Autodesk Inventor part; units mm, degrees
ref_plane "YZ Plane" through (0, 0, 0) normal (1, 0, 0) x (0, 1, 0)
ref_plane "XZ Plane" through (0, 0, 0) normal (0, 1, 0) x (-1, 0, 0)
ref_plane "XY Plane" through (0, 0, 0) normal (0, 0, 1) x (1, 0, 0)
sketch "Sketch1" plane through (0, 0, 0) normal (0, 0, 1) x (1, 0, 0)
  line L0 (9.7407, 1114.2593) -> (159.7407, 1114.2593)
  line L1 (9.7407, 1114.2593) -> (-140.2593, 1114.2593)
  line L2 (-290.2593, 814.2593) -> (-140.2593, 1114.2593)
  line L3 (159.7407, 1114.2593) -> (459.7407, 514.2593)
  line L4 (135.0194, 1074.2593) -> (9.7407, 1074.2593)
  line L5 (9.7407, 1074.2593) -> (-115.5379, 1074.2593)
  line L6 (-115.5379, 1074.2593) -> (-245.5379, 814.2593)
  line L7 (9.7407, 1114.2593) -> (159.7407, 1114.2593)
  line L8 (9.7407, 1114.2593) -> (-140.2593, 1114.2593)
  line L9 (-440.2593, 514.2593) -> (-140.2593, 1114.2593)
  line L10 (159.7407, 1114.2593) -> (309.9483, 813.8441)
  line L11 (135.0194, 1074.2593) -> (9.7407, 1074.2593)
  line L12 (9.7407, 1074.2593) -> (-115.5379, 1074.2593)
  line L13 (-115.5379, 1074.2593) -> (-245.5379, 814.2593)
  line L14 (-245.5379, 814.2593) -> (-290.2593, 814.2593)
  line L15 (265.227, 813.8441) -> (309.9483, 813.8441)
  line L16 (265.227, 813.8441) -> (135.0194, 1074.2593)
  line L17 (415.0194, 514.2593) -> (135.0194, 1074.2593)
  line L18 (-395.5379, 514.2593) -> (-440.2593, 514.2593)
  line L19 (-245.5379, 814.2593) -> (-395.5379, 514.2593)
  line L20 (-440.2593, 514.2593) -> (-395.5379, 514.2593)
  line L21 (415.0194, 514.2593) -> (459.7407, 514.2593)
  point P0 (0, 0)
  dimension "d13" = 300
extrude "Extrusion1" add sketch "Sketch1" along normal blind 40 contours L0 L3 L15 L16 L4 L5 L6 L14 L2 L1
fillet "Fillet2" radius 0.5 1 edges at (200.1232, 944.0517, 0)
fillet "Fillet3" radius 0.5 3 edges at (159.7407, 1114.2593, 20) (84.7407, 1114.2593, 0) (-215.2593, 964.2593, 0)
sketch "Sketch2" plane through (-140.2593, 1114.2593, 0.5) normal (0, 1, 0) x (1, 0, 0)
  line L0 (300.1382, -39.5) -> (300.1382, 0.4472)
  line L1 (300.1382, -19.5) -> (0, -19.5)
  line L2 (0, 0) -> (0, -39.5)
  circle A0 centre (150.0691, -19.5) radius 1.5
  point P0 (140.2593, 0.5)
  point P1 (300.1382, -39)
  point P2 (300.1382, 0)
  point P3 (0, -39)
  dimension "d14" = 3
extrude "Extrusion2" cut sketch "Sketch2" against normal blind 10
extrude "Extrusion3" add sketch "Sketch1" along normal blind 40 contours L3 L21 L17 L15 | L14 L19 L18 L9
sketch "Sketch3" plane through (-140.2593, 1114.2593, 0.5) normal (0, 1, 0) x (1, 0, 0)
  point P0 (140.2593, 0.5)
sketch "Sketch4" plane through (-140.2593, 1114.2593, 0.5) normal (0, 1, 0) x (1, 0, 0)
  circle A0 centre (150.0691, -19.5) radius 1.5
  line L0 (0, 0) -> (299.691, 0)
  line L1 (0, 0) -> (0, -39.5)
  line L2 (299.691, 0) -> (299.691, -39.5)
  line L3 (200.1691, -14.5) -> (225.9691, -14.5)
  line L4 (225.9691, -24.5) -> (200.1691, -24.5)
  arc A1 (225.9691, -24.5) -> (225.9691, -14.5) centre (225.9691, -19.5) ccw
  arc A2 (200.1691, -14.5) -> (200.1691, -24.5) centre (200.1691, -19.5) ccw
  arc A3 (74.1691, -14.5) -> (74.1691, -24.5) centre (74.1691, -19.5) ccw
  line L5 (74.1691, -14.5) -> (99.9691, -14.5)
  line L6 (74.1691, -24.5) -> (99.9691, -24.5)
  arc A4 (99.9691, -24.5) -> (99.9691, -14.5) centre (99.9691, -19.5) ccw
  line L7 (299.691, -39.5) -> (0, -39.5)
  point P0 (140.2593, 0.5)
extrude "Extrusion4" cut sketch "Sketch4" against normal blind 50 contours L3 A1 L4 A2 | L5 A4 L6 A3
sketch "Esboço5" plane through (0, 0, 0) normal (0, 0, 1) x (1, 0, 0)
  line L0 (159.4317, 1114.2593) -> (-140.2593, 1114.2593)
  line L1 (-94.9789, 1114.2593) -> (-94.9789, 897.5465)
  line L2 (-94.9789, 897.5465) -> (-260.935, 897.5465)
  line L3 (-290.2593, 814.2593) -> (-140.2593, 1114.2593)
  line L4 (-250.2227, 877.5465) -> (-250.2227, 857.5465)
  line L5 (265.227, 813.8441) -> (135.0194, 1074.2593)
  line L6 (223.3758, 897.5465) -> (233.3758, 897.5465)
  line L7 (233.3758, 897.5465) -> (233.3758, 882.5465)
  line L8 (-94.9789, 897.5465) -> (445.9224, 897.5465)
  line L9 (268.1798, 897.5465) -> (258.1798, 897.5465)
  line L10 (268.1798, 897.5465) -> (258.1798, 897.5465)
  line L11 (258.1798, 897.5465) -> (258.1798, 882.5465)
  line L12 (258.1798, 882.5465) -> (258.1798, 877.5465)
  line L13 (258.1798, 862.5465) -> (258.1798, 857.5465)
  line L14 (258.1798, 857.5465) -> (258.1798, 852.5465)
  arc A0 (253.1798, 857.5465) -> (263.1798, 857.5465) centre (258.1798, 857.5465) ccw
  arc A1 (263.1798, 877.5465) -> (253.1798, 877.5465) centre (258.1798, 877.5465) ccw
  line L15 (263.1798, 877.5465) -> (263.1798, 857.5465)
  line L16 (253.1798, 857.5465) -> (253.1798, 877.5465)
  line L17 (-248.6157, 897.5465) -> (-293.337, 808.1037)
  line L18 (268.1798, 897.5465) -> (312.835, 808.0707)
  line L19 (459.7407, 514.2593) -> (159.9907, 1113.7593)
  line L20 (-293.337, 808.1037) -> (-248.6157, 808.1037)
  line L21 (-395.5379, 514.2593) -> (-115.5379, 1074.2593)
  line L22 (-248.6157, 808.1037) -> (-258.6157, 808.1037)
  line L23 (-258.6157, 808.1037) -> (-258.6157, 823.1037)
  line L24 (-258.6157, 823.1037) -> (-258.6157, 828.1037)
  line L25 (-258.6157, 848.1037) -> (-258.6157, 853.1037)
  arc A2 (-253.6157, 848.1037) -> (-263.6157, 848.1037) centre (-258.6157, 848.1037) ccw
  arc A3 (-263.6157, 828.1037) -> (-253.6157, 828.1037) centre (-258.6157, 828.1037) ccw
  line L26 (-263.6157, 828.1037) -> (-263.6157, 848.1037)
  line L27 (-253.6157, 848.1037) -> (-253.6157, 828.1037)
  line L28 (-258.6157, 828.1037) -> (-258.6157, 833.1037)
  line L29 (-258.6157, 843.1037) -> (-258.6157, 848.1037)
  line L30 (312.835, 808.0707) -> (268.1137, 808.0707)
  line L31 (135.0194, 1074.2593) -> (415.0194, 514.2593)
  line L32 (268.1137, 808.0707) -> (278.1137, 808.0707)
  line L33 (278.1137, 808.0707) -> (278.1137, 823.0707)
  line L34 (278.1137, 823.0707) -> (278.1137, 828.0707)
  line L35 (278.1137, 848.0707) -> (278.1137, 853.0707)
  arc A4 (283.1137, 848.0707) -> (273.1137, 848.0707) centre (278.1137, 848.0707) ccw
  arc A5 (273.1137, 828.0707) -> (283.1137, 828.0707) centre (278.1137, 828.0707) ccw
  line L36 (273.1137, 848.0707) -> (273.1137, 828.0707)
  line L37 (283.1137, 848.0707) -> (283.1137, 828.0707)
  line L38 (278.1137, 828.0707) -> (278.1137, 833.0707)
  line L39 (278.1137, 843.0707) -> (278.1137, 848.0707)
  line L40 (-238.6157, 882.5465) -> (-238.6157, 862.5465)
  line L41 (-233.6157, 862.5465) -> (-233.6157, 882.5465)
  line L42 (-243.6157, 882.5465) -> (-243.6157, 862.5465)
  line L43 (-248.6157, 897.5465) -> (-238.6157, 897.5465)
  line L44 (-238.6157, 897.5465) -> (-238.6157, 882.5465)
  line L45 (-293.337, 808.1037) -> (-248.6157, 808.1037)
  line L46 (-248.6157, 897.5465) -> (-238.6157, 897.5465)
  line L47 (-238.6157, 897.5465) -> (-238.6157, 882.5465)
  line L48 (-238.6157, 882.5465) -> (-238.6157, 877.5465)
  line L49 (-238.6157, 857.5465) -> (-238.6157, 852.5465)
  arc A6 (-243.6157, 857.5465) -> (-233.6157, 857.5465) centre (-238.6157, 857.5465) ccw
  arc A7 (-233.6157, 877.5465) -> (-243.6157, 877.5465) centre (-238.6157, 877.5465) ccw
  line L50 (-243.6157, 877.5465) -> (-243.6157, 857.5465)
  line L51 (-233.6157, 857.5465) -> (-233.6157, 877.5465)
  line L52 (-238.6157, 877.5465) -> (-238.6157, 872.5465)
  line L53 (-238.6157, 862.5465) -> (-238.6157, 857.5465)
  point P0 (0, 0)
  dimension "d23" = 216.7128
  dimension "d33" = 10
  dimension "d34" = 15
  dimension "d35" = 5
  dimension "d37" = 20
  dimension "d38" = 5
  dimension "d39" = 10
  dimension "d40" = 100
  dimension "d41" = 100
  dimension "d42" = 10
  dimension "d43" = 15
  dimension "d44" = 5
  dimension "d45" = 20
  dimension "d46" = 5
  dimension "d47" = 10
  dimension "d48" = 10
  dimension "d49" = 10
  dimension "d50" = 15
  dimension "d51" = 5
  dimension "d52" = 20
  dimension "d53" = 5
  dimension "d54" = 10
  dimension "d55" = 10
  dimension "d69" = 10
  dimension "d70" = 15
  dimension "d71" = 5
  dimension "d72" = 20
  dimension "d73" = 5
  dimension "d74" = 10
  dimension "d75" = 10
extrude "Extrusão5" cut sketch "Esboço5" along normal mid plane 1000 contours A5 L36 A4 L37 | A1 L15 A0 L16 | A3 L26 A2 L27 | A7 L41 L51 A6 L49 L53 L40 | L40 L53 L49 A6 L50 L42 A7
sketch "Esboço8" plane through (0, 0, 40) normal (0, 0, 1) x (1, 0, 0)
  point P0 (0, 0)
properties part number "Cavalete_Inferior" material "SAE 1010/1020"
Build history of the part. All positions in model axes, mm. A direction names the side the tool comes from. Coordinates: 2 decimals unless noted, no trailing zeros. Order: outer loops, then holes, each group sorted by start corner. A loop starts at its lowest first (then second) coordinate and runs counter-clockwise, first axis right, second up. Notation, with made-up numbers: (54.5, 34) - (68.5, 34) arc R6 cw to (68.5, 42) - close; hole circle Ø1 at (75, 25). An arc over 180 degrees is marked (long way). Put each result on its own line as item: value.
1. Saw through at A-A (z = 31.5). Write the cut outline in (x, y), and give its area (3 significant figures).
Answer sheet:
outline: (-440.26, 514.26) - (-395.54, 514.26) - (-115.54, 1074.26) - (135.02, 1074.26) - (415.02, 514.26) - (459.74, 514.26) - (159.88, 1113.98) arc R0.5 ccw to (159.43, 1114.26) - (-140.26, 1114.26) - close; hole (-263.62, 828.1) arc R5 ccw to (-253.62, 828.1) - (-253.62, 848.1) arc R5 ccw to (-263.62, 848.1) - close; hole (-243.62, 857.55) arc R5 ccw to (-233.62, 857.55) - (-233.62, 877.55) arc R5 ccw to (-243.62, 877.55) - close; hole (253.18, 857.55) arc R5 ccw to (263.18, 857.55) - (263.18, 877.55) arc R5 ccw to (253.18, 877.55) - close; hole (273.11, 828.07) arc R5 ccw to (283.11, 828.07) - (283.11, 848.07) arc R5 ccw to (273.11, 848.07) - close
area: 61,800 mm^2
2. Drop flat-ended pins along their axis: P1, Ø22, axis at y = 836, z = 25, coming from the -X side; P2, Ø1, axis at y = 955, z = 15, coming from the -X side; P3, Ø0.6, axis at x = 265.5, z = 0, coming from the +Y side. Give the stop position or say it passes through.
Answer sheet:
P1: stops at x = -284.89
P2: stops at x = -220.14
P3: stops at y = 903.34
3. Probe line 1 along X through (y, z) = (1111.5, 20); line 2 along X through (y, z) = (869.5, 15.5); line 3 along X through (y, z) = (694, 23.5). List the from-to ranges inside material, lowest first. Write a range as [from, to].
Answer sheet:
line 1: x = [-141.64, -71.09], [-35.29, 8.31], [11.31, 54.91], [90.71, 161.12]
line 2: x = [-262.64, -243.62], [-233.62, -217.92], [237.4, 253.18], [263.18, 282.12]
line 3: x = [-350.39, -305.67], [325.15, 369.87]
4. Saw through at C-C (x = 389.5). Write the cut outline in (y, z), and give its area (3 significant figures).
Answer sheet:
outline: (565.3, 0) - (654.74, 0) - (654.74, 40) - (565.3, 40) - close
area: 3,580 mm^2
5. Saw through at B-B (y = 558.5). Write the cut outline in (x, z), and give its area (3 significant figures).
Answer sheet:
outline: (-418.14, 0) - (-373.42, 0) - (-373.42, 40) - (-418.14, 40) - close; (392.9, 0) - (437.62, 0) - (437.62, 40) - (392.9, 40) - close
area: 3,580 mm^2
6. Tool access for faces 5 (the face through (-253.616, 838, 20)), 6 (the face through (-253.578, 798.179, 19.72)), 7 (the face through (199.401, 945.832, 0.143)), 8 (the face through (73, 1095, 25)): list every direction of +Z, -Z, +X, -X, +Y, -Y with a clear straight run to the whole face (end or side of a thin tool).
Answer sheet:
face 5: +Z, -Z
face 6: +Z, -Z, -Y
face 7: -Z, -Y
face 8: +Y, -Y
7. Saw through at D-D (x = -125.5). Write the cut outline in (y, z), and give its area (3 significant figures).
Answer sheet:
outline: (1054.34, 0) - (1113.76, 0) arc R0.5 ccw to (1114.26, 0.5) - (1114.26, 40) - (1054.34, 40) - close
area: 2,400 mm^2
8. Pull direction Y, two halves, no side cores. Call faces 1 (the face through (307.71, 818.32, 19.72)), 2 (the face through (-243.616, 868, 20)), 3 (the face through (73, 1095, 15)), 4 (the face through (-418, 514.259, 20)): pulls with the +Y half, pulls with the -Y half, needs draft (parallel to the pull), parting line crosses it, or undercut.
Answer sheet:
face 1: pulls with the +Y half
face 2: undercut
face 3: needs draft
face 4: pulls with the -Y half
